```python
from build123d import *

# Parameters (mm, degrees)
F0_W     = 40
F0_H     = 60
F1_DEPTH = 3
F2_R     = 5


with BuildPart() as f1:
    # F0 (on Top) → F1 (new body)
    with BuildSketch(Plane.XY):
        Rectangle(F0_W, F0_H)
        with BuildLine():
            ThreePointArc((-10.9, -20), (-13.6313708499, -21.1313708499), (-12.5, -18.4))
            ThreePointArc((-12.5, -18.4), (-11.3686291501, -18.8686291501), (-10.9, -20))
        make_face(mode=Mode.SUBTRACT)
        with BuildLine():
            ThreePointArc((14.1, -20), (11.3686291501, -21.1313708499), (12.5, -18.4))
            ThreePointArc((12.5, -18.4), (13.6313708499, -18.8686291501), (14.1, -20))
        make_face(mode=Mode.SUBTRACT)
        with BuildLine():
            ThreePointArc((-12.5, 1.6), (-11.3686291501, 1.1313708499), (-10.9, 0))
            ThreePointArc((-10.9, 0), (-11.3686291501, -1.1313708499), (-12.5, -1.6))
            ThreePointArc((-12.5, -1.6), (-14.1, 0), (-12.5, 1.6))
        make_face(mode=Mode.SUBTRACT)
        with BuildLine():
            ThreePointArc((-10.9, 20), (-11.3686291501, 18.8686291501), (-12.5, 18.4))
            ThreePointArc((-12.5, 18.4), (-13.6313708499, 21.1313708499), (-10.9, 20))
        make_face(mode=Mode.SUBTRACT)
        Polygon((6.5, 6), (6.5, 0), (6.5, -6), (-6.5, -6), (-6.5, 0), (-6.5, 6), align=None, mode=Mode.SUBTRACT)
        with BuildLine():
            ThreePointArc((12.5, -1.6), (11.3686291501, -1.1313708499), (10.9, 0))
            ThreePointArc((10.9, 0), (11.3686291501, 1.1313708499), (12.5, 1.6))
            ThreePointArc((12.5, 1.6), (13.6313708499, 1.1313708499), (14.1, 0))
            ThreePointArc((14.1, 0), (13.6313708499, -1.1313708499), (12.5, -1.6))
        make_face(mode=Mode.SUBTRACT)
        with BuildLine():
            ThreePointArc((14.1, 20), (13.6313708499, 18.8686291501), (12.5, 18.4))
            ThreePointArc((12.5, 18.4), (11.3686291501, 21.1313708499), (14.1, 20))
        make_face(mode=Mode.SUBTRACT)
    extrude(amount=F1_DEPTH)

    # F2
    f2_edges = [f1.edges().sort_by_distance(p)[0] for p in [
        (20, -30, 1.5),
        (20, 30, 1.5),
        (-20, -30, 1.5),
        (-20, 30, 1.5),
    ]]
    fillet(f2_edges, radius=F2_R)


solid = f1.part
```
Source: CAD feature listing. Evaluate the final solid. Frame: model axes, mm. A direction names the side the tool comes from. Give positions to 0.01 mm unless a question says otherwise; leave off trailing zeros. Write each loop counter-clockwise with the first axis right and the second up, starting at its lowest first coordinate (ties: lowest second). Pieces come first, ordered by that corner, then holes. Notation, with made-up numbers: (81.5, -5.75) - (94.5, -5.75) arc R16 cw to (94.5, 17.25) - close; hole circle Ø3 at (-30.75, 2.25). An arc over 180 degrees is marked (long way). One line per item, written item: value. Start each with the question number.
Q1. First-contact query: pin 1 Ø4 at (x, y) = (-12.5, 20) entering from +Z. Flat tip, straight axial feed; report the tip coordinate or a pass-through.
Q2. Section query B-B, the plane z = 0.6. Return the cut outline in (x, y), then the cut area to 3 significant figures.
Q3. Draft query along Y for faces 3 (the face through (18, -29, 2)), 4 (the face through (-6.5, 0, 1)), 5 (the face through (0, 7, 3)), 6 (the face through (0, -6, 1)). Return one class per face: +Y half, -Y half, draft (parallel to the pull), parting line (faces both ways), or undercut.
Q4. Section query A-A, the plane x = -1. Return the cut outline in (y, z), then the cut area to 3 significant figures.
Q5. Material intervals for probe 1 along Y at (x, z) = (12.5, 0.8); probe 2 along X at (y, z) = (20, 2); probe 3 along Y at (x, z) = (13, 2), sorted ascending. Write a range as from..to.
Q6. Set-up query: faces 1 (the face through (0, 6, 1)), 2 (the face through (0, 7, 0)). Return all of +Z, -Z, +X, -X, +Y, -Y with unobstructed straight access to the full face (end or side cutting, diameter ignored); none if empty.
Answer:
1. pin 1: stops at z = 3
2. outline: (-20, -25) arc R5 ccw to (-15, -30) - (15, -30) arc R5 ccw to (20, -25) - (20, 25) arc R5 ccw to (15, 30) - (-15, 30) arc R5 ccw to (-20, 25) - close; hole circle Ø3.2 at (-12.5, -20); hole circle Ø3.2 at (-12.5, 0); hole circle Ø3.2 at (-12.5, 20); hole (-6.5, -6) - (6.5, -6) - (6.5, 6) - (-6.5, 6) - close; hole circle Ø3.2 at (12.5, -20); hole circle Ø3.2 at (12.5, 0); hole circle Ø3.2 at (12.5, 20)
2. area: 2,170 mm2
3. face 3: -Y half
3. face 4: undercut
3. face 5: draft
3. face 6: undercut
4. outline: (-30, 0) - (-6, 0) - (-6, 3) - (-30, 3) - close; (6, 0) - (30, 0) - (30, 3) - (6, 3) - close
4. area: 144 mm2
5. probe 1: y = -30..-21.6, -18.4..-1.6, 1.6..18.4, 21.6..30
5. probe 2: x = -20..-14.1, -10.9..10.9, 14.1..20
5. probe 3: y = -30..-21.52, -18.48..-1.52, 1.52..18.48, 21.52..30
6. face 1: +Z, -Z
6. face 2: -Z, +X, -X, +Y, -Y
